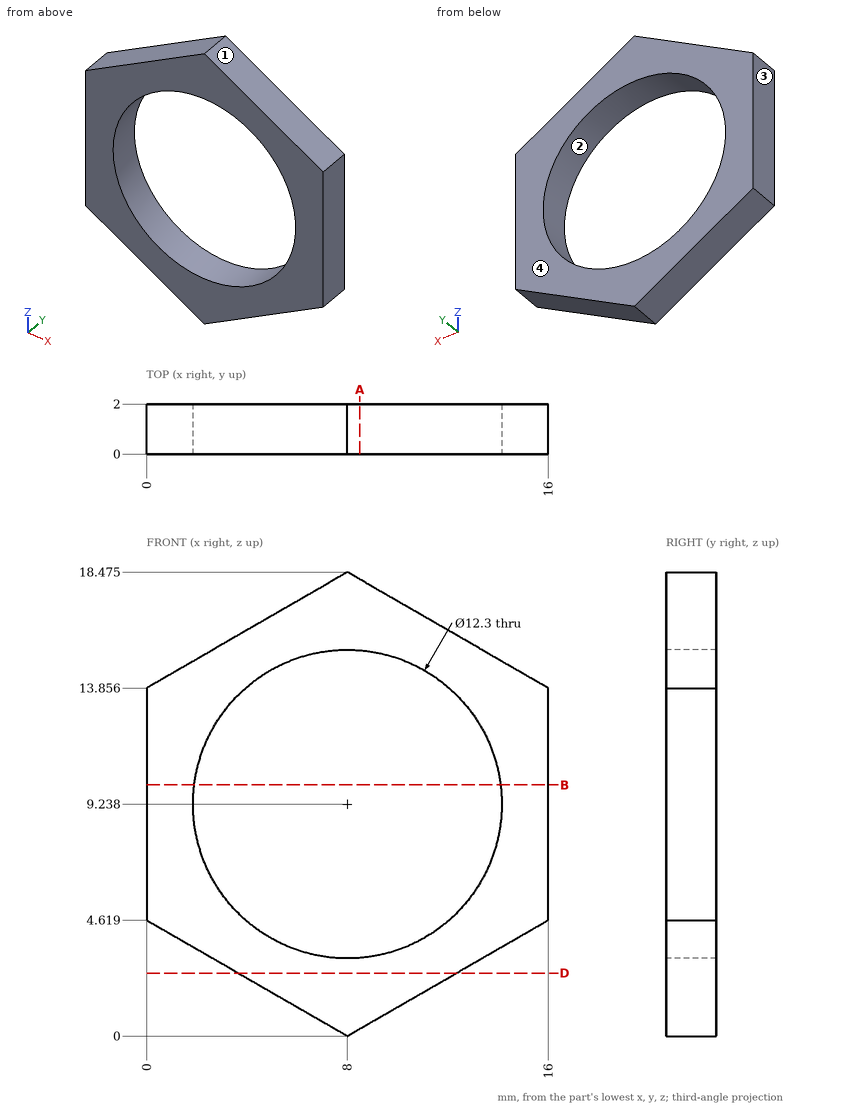
The drawing under review shows one solid part. Ordinate dimensions are in mm from its lowest x, y, z. Round coordinates to 2 decimals unless told otherwise and drop trailing zeros. Write each loop counter-clockwise with the first axis right and the second up, starting at its lowest first coordinate (ties: lowest second). Pieces come first, ordered by that corner, then holes.
(1) Wall thickness on L1, parallel to Z at x = 3.75, y = 1.6 (1 decimal); L2, parallel to X at y = 1.9, z = 13 (1 decimal); L3, parallel to Z at x = 5.25, y = 1.25 (1 decimal): over which ranges is each line inside the solid? List them lowest first.
(2) We need section D-D on z = 2.5. Give the boundary of the cut face in (x, y), and give its area (3 significant figures).
(3) Mouldability with a two-part tool opening along X and no side actions: class the marked faces 1, 2, 3 and 4 as +X half, -X half, draft (parallel to the pull), parting line (faces both ways), or undercut.
(4) We need section A-A on x = 8.5. Give the boundary of the cut face in (y, z).
(5) We need section B-B on z = 10. Give the boundary of the cut face in (x, y).
Findings below:
1. L1: z = 2.5 to 4.8, 13.7 to 16
1. L2: x = 0 to 3.1, 12.9 to 16
1. L3: z = 1.6 to 3.7, 14.7 to 16.9
2. outline: (3.67, 0) - (12.33, 0) - (12.33, 2) - (3.67, 2) - close
2. area: 17.3 mm2
3. face 1: +X half
3. face 2: undercut
3. face 3: -X half
3. face 4: draft
4. outline: (0, 0.29) - (2, 0.29) - (2, 3.11) - (0, 3.11) - close; (0, 15.37) - (2, 15.37) - (2, 18.19) - (0, 18.19) - close
5. outline: (0, 0) - (1.9, 0) - (1.9, 2) - (0, 2) - close; (14.1, 0) - (16, 0) - (16, 2) - (14.1, 2) - close
